from build123d import *

# Parameters (mm, degrees)
SKETCH1_R      = 3.175
EXTRUDE1_DEPTH = 38.1
CHAMFER1_SIZE  = 0.15875


with BuildPart() as part:
    # Sketch1 → Extrude1 (new, symmetric)
    with BuildSketch(Plane.XY):
        with Locations(Location((0, 0, 0), (0, 0, 180))):
            Circle(SKETCH1_R)
    extrude(amount=EXTRUDE1_DEPTH, both=True)

    # Sketch6 → Cut-Revolve2 (revolve, cut)
    with BuildSketch(Plane(origin=(0, 0, 0), x_dir=(0, 0, -1), z_dir=(1, 0, 0)), mode=Mode.PRIVATE) as cut_revolve2_sk:
        Polygon((-36.5125, 3.175), (-36.5125, 1.5875), (-35.7759, 1.5875), (-35.7759, 3.175), (-29.4259, 3.175), (-29.4259, 1.5875), (-28.6893, 1.5875), (-28.6893, 3.175), (-22.3393, 3.175), (-22.3393, 1.5875), (-21.6027, 1.5875), (-21.6027, 3.175), (-15.2527, 3.175), (-15.2527, 1.5875), (-14.5161, 1.5875), (-14.5161, 3.175), (-8.1661, 3.175), (-8.1661, 1.5875), (-7.4295, 1.5875), (-7.4295, 3.175), (28.6893, 3.175), (28.6893, 1.5875), (29.4259, 1.5875), (29.4259, 3.175), (35.7759, 3.175), (35.7759, 1.5875), (36.5125, 1.5875), (36.5125, 3.175), (38.1, 3.175), (38.1, 5.715), (-38.1, 5.715), (-38.1, 3.175), align=None)
    revolve(cut_revolve2_sk.sketch.rotate(Axis((0, 0, 38.1), (0, 0, -1)), 270), axis=Axis((0, 0, 38.1), (0, 0, -1)), mode=Mode.SUBTRACT)

    # Chamfer1
    chamfer1_edges = [part.edges().sort_by_distance(p)[0] for p in [
        (3.175, 0, -38.1),
        (3.175, 0, 38.1),
    ]]
    chamfer(chamfer1_edges, length=CHAMFER1_SIZE)


solid = part.part
CAD build for the part. Positions are in the model's coordinates, mm. A direction names the side the tool comes from. Round coordinates to 2 decimals unless told otherwise and drop trailing zeros. Loops run counter-clockwise (first coordinate to the right, second up) from the corner with the lowest first, then second, coordinate; pieces in that order, holes last.
(1) Wall check: line 1 along X through (y, z) = (-2.75, 30.5); line 2 along X through (y, z) = (1, 34). Give the ranges that are in metal, low to high.
(2) Cut at A-A (z = 16.5). Give the cut face in (x, y) (3 decimals).
(3) Drop a flat-ended pin along its axis: pin 1 (1 mm diameter, centred on y = -2, z = 3.5, fed in from -X). Give the stop position or say it passes through.
(4) Two-plate mould, pull along X, no slides. Class faces 3 (the cylindrical face through (1.26, -0.966, 36.139)), 4 (the flat face through (1.4, -1.4, 14.516)): +X half, -X half, draft (parallel to the pull), parting line (faces both ways), or undercut.
(5) Which spindle directions (+Z, -Z, +X, -X, +Y, -Y) get a long thin tool onto all of the face, cutting with end or side? Do faces 1 (the cylindrical face through (1.26, -0.966, 7.793)), 2 (the cylindrical face through (-1.5, 2.8, 37.2)). Say none if no direction does.
Findings below:
1. line 1: x = -1.59 to 1.59
1. line 2: x = -3.01 to 3.01
2. outline: circle Ø6.35 at (0, 0)
3. pin 1: stops at x = -2.8
4. face 3: parting line
4. face 4: draft
5. face 1: none
5. face 2: +Z, -Z
